The figure shows three views and two pictorial views of one solid part (mm, origin at its lowest corner). Answer the questions. A direction names the side the tool comes from. Coordinates: 2 decimals unless noted, no trailing zeros. Order: outer loops, then holes, each group sorted by start corner. A loop starts at its lowest first (then second) coordinate and runs counter-clockwise, first axis right, second up.
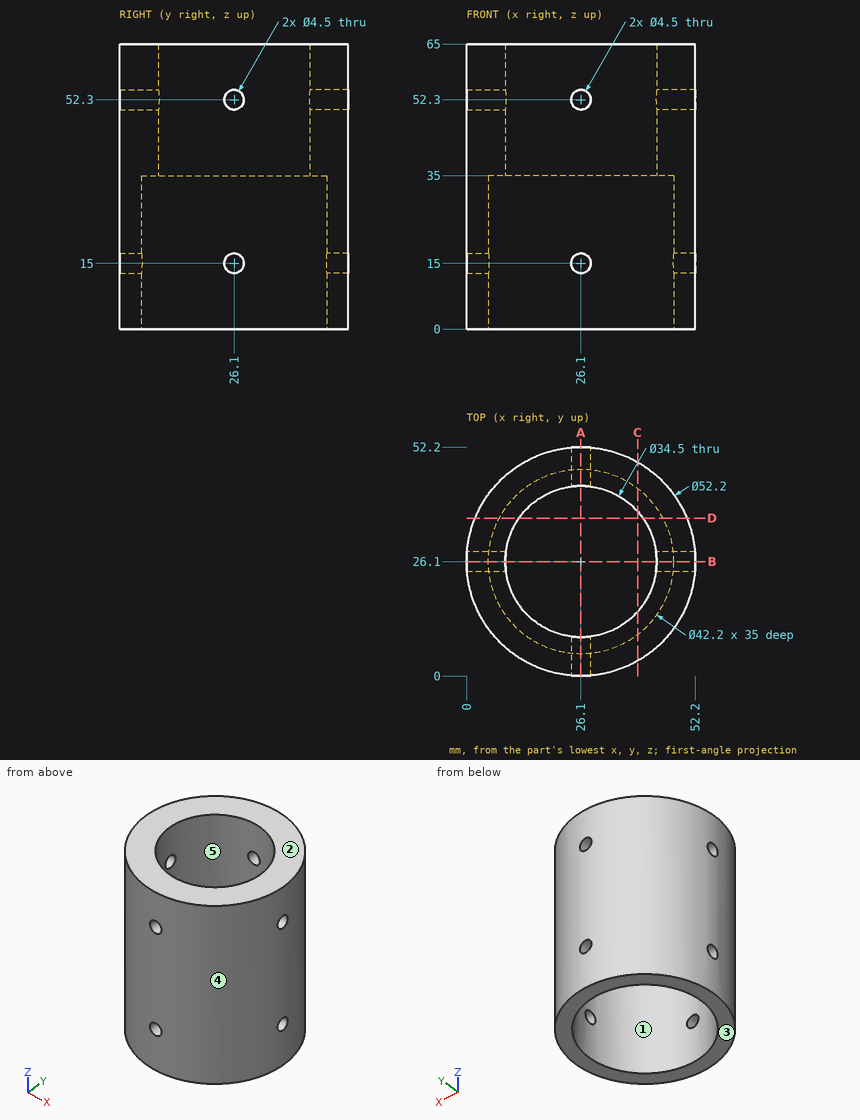
Q1. The part is cut by section C-C, the plane x = 39. Determine the outline of the cut face in (y, z), then the cut area to 3 significant figures.
Q2. Each of these flat-tipped pins is pushed along its axis until it touches: P1, Ø8, axis at y = 39, z = 32, coming from the +X side; P2, Ø4, axis at x = 26.1, z = 15, coming from the -Y side; P3, Ø4, axis at y = 7, z = 12.5, coming from the +X side; P4, Ø1.5, axis at x = 37, z = 19, coming from the -Y side. Where does it stop, or does it pass through?
Q3. The part is cut by section D-D, the plane y = 36. Determine the outline of the cut face in (x, z), then the cut area to 3 significant figures.
Q4. Which of the six approach directions +Z, -Z, +X, -X, +Y, -Y give full straight-line access (tool end or side, diameter ignored) to the marked faces 1 and 2?
Q5. The part is cut by section A-A, the plane x = 26.1. Determine the outline of the cut face in (y, z), then the cut area to 3 significant figures.
Q6. Straight lines are drawn through the part: L1, parallel to Y at x = 26.1, z = 56; L2, parallel to Y at x = 26, z = 10; L3, parallel to X at y = 23, z = 4. For each, find the intervals that lie inside material, in ascending order.
Q7. Determine the mould class of the marked faces 3, 4 and 5 for opening direction Y: +Y half, -Y half, draft (parallel to the pull), parting line (faces both ways), or undercut.
Computed values:
1. outline: (3.41, 0) - (9.4, 0) - (9.4, 35) - (14.65, 35) - (14.65, 65) - (3.41, 65) - close; (37.55, 35) - (42.8, 35) - (42.8, 0) - (48.79, 0) - (48.79, 65) - (37.55, 65) - close
1. area: 1,090 mm2
2. P1: stops at x = 50.64
2. P2: passes through
2. P3: stops at x = 45.82
2. P4: stops at y = 2.05
3. outline: (1.95, 0) - (7.47, 0) - (7.47, 35) - (11.97, 35) - (11.97, 65) - (1.95, 65) - close; (40.23, 35) - (44.73, 35) - (44.73, 0) - (50.25, 0) - (50.25, 65) - (40.23, 65) - close
3. area: 988 mm2
4. face 1: -Z
4. face 2: +Z, +X, -X, +Y, -Y
5. outline: (0, 0) - (5, 0) - (5, 12.75) - (0, 12.75) - close; (0, 17.25) - (5, 17.25) - (5, 35) - (8.85, 35) - (8.85, 50.05) - (0, 50.05) - close; (0, 54.55) - (8.85, 54.55) - (8.85, 65) - (0, 65) - close; (43.35, 35) - (47.2, 35) - (47.2, 17.25) - (52.2, 17.25) - (52.2, 50.05) - (43.35, 50.05) - close; (43.35, 54.55) - (52.2, 54.55) - (52.2, 65) - (43.35, 65) - close; (47.2, 0) - (52.2, 0) - (52.2, 12.75) - (47.2, 12.75) - close
5. area: 756 mm2
6. L1: y = 0 to 8.85, 43.35 to 52.2
6. L2: y = 0 to 5, 47.2 to 52.2
6. L3: x = 0.18 to 5.23, 46.97 to 52.02
7. face 3: draft
7. face 4: parting line
7. face 5: undercut
